from build123d import *

# Parameters (mm, degrees)
BOSS_EXTRUDE1_DEPTH      = 5.08
SKETCH2_W                = 63.5
SKETCH2_H                = 7
CUT_EXTRUDE1_DEPTH       = 0.635
SKETCH3_W                = 6.35
SKETCH3_H                = 6.35
SKETCH3_R                = 1.5875
BOSS_EXTRUDE2_DEPTH      = 3.81
CHAMFER1_SIZE            = 0.635
CHAMFER1_OF_MIRROR1_SIZE = 0.635
SKETCH6_R                = 2.413
CUT_EXTRUDE2_DEPTH       = 103.813663911
SKETCH7_R                = 1.20015
CUT_EXTRUDE3_DEPTH       = 103.854835627


with BuildPart() as part:
    # Sketch1 → Boss-Extrude1 (new body)
    with BuildSketch(Plane.XY):
        with BuildLine():
            Line((-35.352091015, 31.75), (-42.972091015, 31.75))
            Line((-42.972091015, 31.75), (-42.972091015, 17.78))
            Line((-42.972091015, 17.78), (-56.942091015, 17.78))
            Line((-56.942091015, 17.78), (-56.942091015, 12.7))
            Line((-56.942091015, 12.7), (-83.612091015, 12.7))
            Line((-83.612091015, 12.7), (-83.612091015, 15.875))
            Line((-83.612091015, 15.875), (-97.582091015, 15.875))
            Line((-97.582091015, 15.875), (-97.582091015, -15.875))
            Line((-97.582091015, -15.875), (-83.612091015, -15.875))
            Line((-83.612091015, -15.875), (-83.612091015, -12.7))
            Line((-83.612091015, -12.7), (-56.942091015, -12.7))
            Line((-56.942091015, -12.7), (-56.942091015, -17.78))
            Line((-56.942091015, -17.78), (-42.972091015, -17.78))
            Line((-42.972091015, -17.78), (-42.972091015, -31.75))
            Line((-42.972091015, -31.75), (-35.352091015, -31.75))
            ThreePointArc((-35.352091015, -31.75), (-28.422412943, 0), (-35.352091015, 31.75))
        make_face()
    extrude(amount=BOSS_EXTRUDE1_DEPTH)

    # Sketch2 → Cut-Extrude1 (cut)
    with BuildSketch(Plane.XY.offset(5.08)):
        with Locations((-59.482091015, 0)):
            Rectangle(SKETCH2_W, SKETCH2_H)
    extrude(amount=-CUT_EXTRUDE1_DEPTH, mode=Mode.SUBTRACT)

    # Sketch3 → Boss-Extrude2 (add)
    with BuildSketch(Plane.ZY.offset(97.582091015)):
        with Locations((8.255, 12.7)):
            Rectangle(SKETCH3_W, SKETCH3_H)
        with Locations((8.255, 12.7)):
            Circle(SKETCH3_R, mode=Mode.SUBTRACT)
    boss_extrude2 = extrude(amount=-BOSS_EXTRUDE2_DEPTH)

    # Chamfer1
    chamfer1_edges = [part.edges().sort_by_distance(p)[0] for p in [
        (-95.677091015, 9.525, 11.43),
        (-95.677091015, 15.875, 11.43),
    ]]
    chamfer(chamfer1_edges, length=CHAMFER1_SIZE)

    # Mirror1: Boss-Extrude2 across plane
    add(boss_extrude2.mirror(Plane.ZX))

    # Chamfer1 of Mirror1
    chamfer1_of_mirror1_edges = [part.edges().sort_by_distance(p)[0] for p in [
        (-95.677091015, -9.525, 11.43),
        (-95.677091015, -15.875, 11.43),
    ]]
    chamfer(chamfer1_of_mirror1_edges, length=CHAMFER1_OF_MIRROR1_SIZE)

    # Sketch6 → Cut-Extrude2 (cut, through all)
    with BuildSketch(Plane.XY.offset(5.08)):
        with Locations((-37.892091015, 22.86)):
            Circle(SKETCH6_R)
        with Locations((-37.892091015, 10.16)):
            Circle(SKETCH6_R)
        with Locations(Location((-37.892091015, -10.16, 0), (0, 0, 180))):
            Circle(SKETCH6_R)
        with Locations(Location((-37.892091015, -22.86, 0), (0, 0, 180))):
            Circle(SKETCH6_R)
    extrude(amount=-CUT_EXTRUDE2_DEPTH, mode=Mode.SUBTRACT)

    # Sketch7 → Cut-Extrude3 (cut, through all)
    with BuildSketch(Plane.XY.offset(4.445)):
        with Locations((-83.731471015, 0)):
            Circle(SKETCH7_R)
        with Locations((-68.745471015, 0)):
            Circle(SKETCH7_R)
        with Locations((-53.759471015, 0)):
            Circle(SKETCH7_R)
        with Locations((-38.773471015, 0)):
            Circle(SKETCH7_R)
    extrude(amount=-CUT_EXTRUDE3_DEPTH, mode=Mode.SUBTRACT)


solid = part.part
Can you work these out from the model? Positions are in its coordinate system, mm. A direction names the side the tool comes from. Coordinates: 2 decimals unless noted, no trailing zeros. Write each loop counter-clockwise with the first axis right and the second up, starting at its lowest first coordinate (ties: lowest second). Pieces come first, ordered by that corner, then holes. Notation, with made-up numbers: (25, 39) -> (36, 39) arc R31 cw to (36, 63) -> close; hole circle Ø5 at (14, 9.5). An arc over 180 degrees is marked (long way). Write each question's results on one line, items separated by ' | '. Start each with the question number.
Q1. We'd pull the mould along Y, two halves only. Please class faces 1 (the face through (-39, 31.75, 3)), 2 (the face through (-54.71, -0.73, 2.25)), 3 (the face through (-83.612, -14, 3)): +Y half, -Y half, draft (parallel to the pull), parting line (faces both ways), or undercut.
Q2. If I drill on probe 1 along Y at (x, z) = (-40, 5); probe 2 along Z at (x, y) = (-36, -26); probe 3 along X at (y, z) = (-10.16, 1.6), over which ranges is the centre line in solid material (lowest first)?
Q3. On a 3-axis mill with a long thin cutter (end or side, diameter ignored), from which of +Z, -Z, +X, -X, +Y, -Y can I reach the whole of each face in a straight line? I mean faces 4 (the face through (-42.972, 25, 3)), 5 (the face through (-96, 9.525, 8)), 6 (the face through (-70, -12.7, 3)). Say none if no direction works.
Q4. Imagine slicing it at B-B (x = -68.5). Write out the boundary of the cut face in (y, z) (3 decimals), then the cut area to 3 significant figures.
Q5. Imagine slicing it at D-D (y = -22.86). Write out the boundary of the cut face in (x, z).
Q6. I'm going to push flat-ended pins straight in: pin 1 (4.5 mm diameter, centred on x = -37.89, y = 22.86, fed in from -Z); pin 2 (3 mm diameter, centred on x = -91.5, z = 4, fed in from -Y) (3 decimals); pin 3 (1 mm diameter, centred on y = 21.5, z = 1.5, fed in from -X); pin 4 (2.5 mm diameter, centred on x = -50, z = 2.5, fed in from -Y). Where does each tip first touch, or does it pass through?
Q7. Imagine slicing it at C-C (x = -49). Write out the boundary of the cut face in (y, z) (3 decimals), then the cut area to 3 significant figures.
Q8. Imagine slicing it at A-A (z = 9). Write out the boundary of the cut face in (x, y) (3 decimals).
Taken from the geometry:
1) face 1: +Y half | face 2: undercut | face 3: draft
2) probe 1: y = -31.75 to -24.03, -21.69 to -11.33, -8.99 to -3.5, 3.5 to 8.99, 11.33 to 21.69, 24.03 to 31.75 | probe 2: z = 0 to 5.08 | probe 3: x = -97.58 to -40.31, -35.48 to -29.1
3) face 4: +Z, -Z, -X, +Y | face 5: +Z, +X, -X | face 6: +Z, -Z, -Y
4) outline: (-12.7, 0) -> (-1.175, 0) -> (-1.175, 4.445) -> (-3.5, 4.445) -> (-3.5, 5.08) -> (-12.7, 5.08) -> close; (1.175, 0) -> (12.7, 0) -> (12.7, 5.08) -> (3.5, 5.08) -> (3.5, 4.445) -> (1.175, 4.445) -> close | area: 114 mm^2
5) outline: (-42.97, 0) -> (-40.31, 0) -> (-40.31, 5.08) -> (-42.97, 5.08) -> close; (-35.48, 0) -> (-31.93, 0) -> (-31.93, 5.08) -> (-35.48, 5.08) -> close
6) pin 1: passes through | pin 2: stops at y = -15.875 | pin 3: stops at x = -42.97 | pin 4: stops at y = -17.78
7) outline: (-17.78, 0) -> (17.78, 0) -> (17.78, 5.08) -> (3.5, 5.08) -> (3.5, 4.445) -> (-3.5, 4.445) -> (-3.5, 5.08) -> (-17.78, 5.08) -> close | area: 176 mm^2
8) outline: (-97.582, -15.875) -> (-93.772, -15.875) -> (-93.772, -14.102) -> (-97.582, -14.102) -> close; (-97.582, -11.298) -> (-93.772, -11.298) -> (-93.772, -9.525) -> (-97.582, -9.525) -> close; (-97.582, 9.525) -> (-93.772, 9.525) -> (-93.772, 11.298) -> (-97.582, 11.298) -> close; (-97.582, 14.102) -> (-93.772, 14.102) -> (-93.772, 15.875) -> (-97.582, 15.875) -> close
